from build123d import *

# Parameters (mm, degrees)
SKETCH1_W           = 50.8
SKETCH1_H           = 50.8
BOSS_EXTRUDE1_DEPTH = 2.54
CUT_EXTRUDE1_DEPTH  = 3.54


with BuildPart() as part:
    # Sketch1 → Boss-Extrude1 (new body)
    with BuildSketch(Plane(origin=(0, 0, 0), x_dir=(1, 0, 0), z_dir=(0, 1, 0))):
        Rectangle(SKETCH1_W, SKETCH1_H)
    extrude(amount=BOSS_EXTRUDE1_DEPTH)

    # Sketch2 → Cut-Extrude1 (cut, through all)
    with BuildSketch(Plane.XZ):
        with BuildLine():
            Line((-4.759535744, 4.759535744), (-2.499599665, 17.278722247))
            ThreePointArc((-2.499599665, 17.278722247), (0, 19.3675), (2.499599665, 17.278722247))
            Line((2.499599665, 17.278722247), (4.759535744, 4.759535744))
            Line((4.759535744, 4.759535744), (17.278722247, 2.499599665))
            ThreePointArc((17.278722247, 2.499599665), (19.3675, 0), (17.278722247, -2.499599665))
            Line((17.278722247, -2.499599665), (4.759535744, -4.759535744))
            Line((4.759535744, -4.759535744), (2.499599665, -17.278722247))
            ThreePointArc((2.499599665, -17.278722247), (0, -19.3675), (-2.499599665, -17.278722247))
            Line((-2.499599665, -17.278722247), (-4.759535744, -4.759535744))
            Line((-4.759535744, -4.759535744), (-17.278722247, -2.499599665))
            ThreePointArc((-17.278722247, -2.499599665), (-19.3675, 0), (-17.278722247, 2.499599665))
            Line((-17.278722247, 2.499599665), (-4.759535744, 4.759535744))
        make_face()
    extrude(amount=-CUT_EXTRUDE1_DEPTH, mode=Mode.SUBTRACT)


solid = part.part
CAD build for the part. Positions are in the model's coordinates, mm. A direction names the side the tool comes from. Coordinates: 2 decimals unless noted, no trailing zeros. Write each loop counter-clockwise with the first axis right and the second up, starting at its lowest first coordinate (ties: lowest second). Pieces come first, ordered by that corner, then holes. Notation, with made-up numbers: (-15.75, -28.75) - (-1.75, -28.75) arc R20 cw to (-1.75, -22.75) - close; hole circle Ø11 at (49, 10). An arc over 180 degrees is marked (long way). Use a Markdown table: item, result. Add a question column.
Item 1: Band-saw the part on C-C, the plane x = 6.5. Give the cut face in (y, z).
Item 2: 3-axis set-ups, long thin cutter, end or side, ignore diameter. For faces 1 (the face through (10.931, 1.252, 3.645)), 2 (the face through (5, 2.54, -6)): which of +Z, -Z, +X, -X, +Y, -Y reach the whole face in a straight line?
Item 3: Band-saw the part on A-A, the plane z = 14. Give the cut face in (x, y), and give its area (3 significant figures).
Item 4: Drill centre lines: L1, parallel to Z at x = 0, y = 2.1; L2, parallel to Z at x = -16.5, y = 0.85; L3, parallel to X at y = 2.05, z = 5. Where is each one in solid material? Low to high. Write a range as from..to.
Item 5: Band-saw the part on B-B, the plane y = 1.2. Give the cut face in (x, z).
Item 6: Mould opens along X. For faces 3 (the face through (3.614, 1.252, 11.107)), 4 (the face through (25.4, 1, 0)), 5 (the face through (0, 1, 25.4)) say: pulls with the +X half, pulls with the -X half, needs draft (parallel to the pull), parting line crosses it, or undercut.
Numbers:
| question | item | result |
|---|---|---|
| 1 | outline | (0, -25.4) - (2.54, -25.4) - (2.54, -4.45) - (0, -4.45) - close; (0, 4.45) - (2.54, 4.45) - (2.54, 25.4) - (0, 25.4) - close |
| 2 | face 1 | +Y, -Y |
| 2 | face 2 | +Z, -Z, +X, -X, +Y |
| 3 | outline | (-25.4, 0) - (-3.09, 0) - (-3.09, 2.54) - (-25.4, 2.54) - close; (3.09, 0) - (25.4, 0) - (25.4, 2.54) - (3.09, 2.54) - close |
| 3 | area | 113 mm2 |
| 4 | L1 | -25.4..-19.37, 19.37..25.4 |
| 4 | L2 | -25.4..-2.64, 2.64..25.4 |
| 4 | L3 | -25.4..-4.72, 4.72..25.4 |
| 5 | outline | (-25.4, -25.4) - (25.4, -25.4) - (25.4, 25.4) - (-25.4, 25.4) - close; hole (-17.28, -2.5) - (-4.76, -4.76) - (-2.5, -17.28) arc R2.54 ccw to (2.5, -17.28) - (4.76, -4.76) - (17.28, -2.5) arc R2.54 ccw to (17.28, 2.5) - (4.76, 4.76) - (2.5, 17.28) arc R2.54 ccw to (-2.5, 17.28) - (-4.76, 4.76) - (-17.28, 2.5) arc R2.54 ccw to start |
| 6 | face 3 | undercut |
| 6 | face 4 | pulls with the +X half |
| 6 | face 5 | needs draft |
